from build123d import *

# Parameters (mm, degrees)
F0_W     = 23
F0_H     = 23
F0_R     = 8.5
F1_DEPTH = 0.6
F3_DEPTH = 9.6
F4_W     = 2.6
F4_H     = 2.6
F4_R     = 0.6
F5_DEPTH = 4
F6_W     = 8
F6_H     = 3
F7_DEPTH = 1.4
F8_R     = 1


with BuildPart() as f1:
    # F0 (on Top) → F1 (new body, symmetric)
    with BuildSketch(Plane.XY):
        with Locations((-11.5, 11.5)):
            Rectangle(F0_W, F0_H)
        Polygon((0, -10.131208), (0, 0), (-23, 0), (-23, -23), (0, -23), (0, -15.231208), (-2.55, -15.231208), (-2.55, -10.131208), align=None)
        with Locations((-13, -12.9)):
            Circle(F0_R, mode=Mode.SUBTRACT)
        with Locations((11.5, 11.5)):
            Rectangle(F0_W, F0_H)
        Polygon((23, 0), (0, 0), (0, -10.131208), (2.55, -10.131208), (2.55, -15.231208), (0, -15.231208), (0, -23), (23, -23), align=None)
        with Locations((13, -12.9)):
            Circle(F0_R, mode=Mode.SUBTRACT)
    extrude(amount=F1_DEPTH, both=True)

    # F2 (on face) → F3 (join)
    with BuildSketch(Plane.XY.offset(0.6)):
        Polygon((-23, 23), (0, 23), (0, 24.2), (-24.2, 24.2), (-24.2, -24.2), (0, -24.2), (0, -23), (-23, -23), align=None)
        Polygon((0, 23), (23, 23), (23, -23), (0, -23), (0, -24.2), (24.2, -24.2), (24.2, 24.2), (0, 24.2), align=None)
    extrude(amount=-F3_DEPTH)

    # F4 (on face) → F5 (join)
    with BuildSketch(Plane(origin=(0, 0, -0.6), x_dir=(1, 0, 0), z_dir=(0, 0, -1))):
        with Locations((21.7, 21.7)):
            Rectangle(F4_W, F4_H)
        with Locations((21.7, 21.7)):
            Circle(F4_R, mode=Mode.SUBTRACT)
        with Locations((-21.7, 21.7)):
            Rectangle(F4_W, F4_H)
        with Locations((-21.7, 21.7)):
            Circle(F4_R, mode=Mode.SUBTRACT)
        with Locations((-21.7, 4.7)):
            Rectangle(F4_W, F4_H)
        with Locations((-21.7, 4.7)):
            Circle(F4_R, mode=Mode.SUBTRACT)
        with Locations((21.7, 4.7)):
            Rectangle(F4_W, F4_H)
        with Locations((21.7, 4.7)):
            Circle(F4_R, mode=Mode.SUBTRACT)
    extrude(amount=F5_DEPTH)

    # F6 (on face) → F7 (cut)
    with BuildSketch(Plane(origin=(-24.2, 0, 0), x_dir=(0, -1, 0), z_dir=(-1, 0, 0))):
        with Locations((-14.2, -2.3)):
            Rectangle(F6_W, F6_H)
    extrude(amount=-F7_DEPTH, mode=Mode.SUBTRACT)

    # F8
    f8_edges = [f1.edges().sort_by_distance(p)[0] for p in [
        (24.2, 0, 0.6),
        (-24.2, 0, 0.6),
        (0, -24.2, 0.6),
        (0, 24.2, 0.6),
        (24.2, -24.2, -4.2),
        (24.2, 24.2, -4.2),
        (-24.2, -24.2, -4.2),
        (-24.2, 24.2, -4.2),
    ]]
    fillet(f8_edges, radius=F8_R)


solid = f1.part
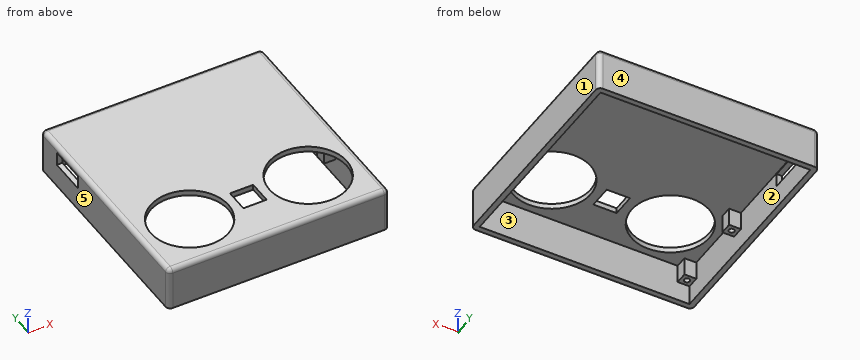
Build history of the part. All positions in model axes, mm. Face numbers are marked on the shaded views. A direction names the side the tool comes from. Give positions to 0.01 mm unless a question says otherwise; leave off trailing zeros. Write each loop counter-clockwise with the first axis right and the second up, starting at its lowest first coordinate (ties: lowest second). Pieces come first, ordered by that corner, then holes. Notation, with made-up numbers: (-2, 56.5) - (50, 56.5) arc R16 cw to (50, 76.5) - close; hole circle Ø7 at (4, 14). An arc over 180 degrees is marked (long way). Use one line per item in the form item = value. Start each with the question number.
1. Band-saw the part on A-A on x = 13. Write the cut outline in (y, z).
2. Band-saw the part on D-D on z = -6. Write the cut outline in (x, y).
3. Band-saw the part on B-B on y = -12.9. Write the cut outline in (x, z), plus the area to 3 significant figures.
4. Probe line 1 (Y direction, x = -21.7, z = -2.5); line 2 (X direction, y = -21.7, z = -2); line 3 (Y direction, x = -13, z = -0.3). List the from-to ranges inside material, lowest first. Write a range as [from, to].
5. Drop flat-ended pins along their axis: pin 1 Ø1.5 at (x, y) = (12.5, 6) entering from -Z; pin 2 Ø1.3 at (x, y) = (21, -21) entering from -Z; pin 3 Ø1.3 at (x, y) = (-24, 14) entering from +Z; pin 4 Ø0.6 at (x, z) = (-23.5, -2.5) entering from +Y. Give the stop position or say it passes through.
6. 3-axis set-ups, long thin cutter, end or side, ignore diameter. For the marked faces 1 and 2: which of +Z, -Z, +X, -X, +Y, -Y reach the whole face in a straight line?
7. Band-saw the part on C-C on z = -1.5. Count the separate pieces of the cut face and the enclosed holes in it, plus the area to 3 significant figures.
8. Two-plate mould, pull along Y, no slides. Class the marked faces 3, 4 and 5: released by +Y, released by -Y, zero draft, split by the parting line, or undercut.
Conclusion:
q1.outline = (-24.2, -9) - (-23, -9) - (-23, -0.6) - (-21.4, -0.6) - (-21.4, 0.6) - (-23.2, 0.6) arc R1 ccw to (-24.2, -0.4) - close; (-4.4, -0.6) - (23, -0.6) - (23, -9) - (24.2, -9) - (24.2, -0.4) arc R1 ccw to (23.2, 0.6) - (-4.4, 0.6) - close
q2.outline = (-24.2, -23.2) arc R1 ccw to (-23.2, -24.2) - (23.2, -24.2) arc R1 ccw to (24.2, -23.2) - (24.2, 23.2) arc R1 ccw to (23.2, 24.2) - (-23.2, 24.2) arc R1 ccw to (-24.2, 23.2) - close; hole (-23, -23) - (23, -23) - (23, 23) - (-23, 23) - close
q3.outline = (-24.2, -9) - (-23, -9) - (-23, -0.6) - (-21.5, -0.6) - (-21.5, 0.6) - (-23.2, 0.6) arc R1 ccw to (-24.2, -0.4) - close; (-4.5, -0.6) - (-2.55, -0.6) - (-2.55, 0.6) - (-4.5, 0.6) - close; (2.55, -0.6) - (4.5, -0.6) - (4.5, 0.6) - (2.55, 0.6) - close; (21.5, -0.6) - (23, -0.6) - (23, -9) - (24.2, -9) - (24.2, -0.4) arc R1 ccw to (23.2, 0.6) - (21.5, 0.6) - close
q3.area = 30.9 mm²
q4.line_1 = [-24.2, -22.3], [-21.1, -20.4], [-6, -5.3], [-4.1, -3.4], [23, 24.2]
q4.line_2 = [-24.2, -22.3], [-21.1, -20.4], [20.4, 21.1], [22.3, 24.2]
q4.line_3 = [-24.19, -21.4], [-4.4, 24.19]
q5.pin_1 = -0.6
q5.pin_2 = -4.6
q5.pin_3 = 0.59
q5.pin_4 = 24.2
q6.face_1 = +Z, -Z, +X, +Y, -Y
q6.face_2 = -Z
q7.separate_pieces = 1
q7.enclosed_holes = 4
q7.area = 239 mm²
q8.face_3 = undercut
q8.face_4 = released by +Y
q8.face_5 = zero draft
